```python
from build123d import *

# Parameters (mm, degrees)
F0_W     = 155.2556827664
F0_H     = 118.4387393296
F1_DEPTH = 57.1
F3_D     = 4.2
F4_R     = 5
F5_SIZE  = 5


with BuildPart() as f1:
    # F0 (on Front) → F1 (new body)
    with BuildSketch(Plane.XZ):
        with Locations((10.389957577, 21.1075376719)):
            Rectangle(F0_W, F0_H)
    extrude(amount=F1_DEPTH)

    # F3 (through all)
    with Locations(Plane(origin=(0, 0, 0), x_dir=(-1, 0, 0), z_dir=(0, 1, 0))):
        with Locations((-35.4269519448, 45.1725050807), (36.4308133721, 45.1725050807), (36.4308133721, 11.5158585832), (-35.4269519448, 11.5158585832)):
            Hole(F3_D / 2)

    # F4
    f4_edges = [f1.edges().sort_by_distance(p)[0] for p in [
        (-67.237884, -28.55, 80.326907),
    ]]
    fillet(f4_edges, radius=F4_R)

    # F5
    f5_edges = [f1.edges().sort_by_distance(p)[0] for p in [
        (88.017799, -28.55, 80.326907),
    ]]
    chamfer(f5_edges, length=F5_SIZE)


solid = f1.part
```
Here's how the part is built. I have some questions about the finished solid (model axes, mm). Coordinates: 2 decimals unless noted, no trailing zeros. Answer as CSV lines item,"result". Start each with the question number.
Q1. I need wall thicknesses on probe 1 along Z at (x, y) = (-35, -24.5). Which ranges of the line are inside material? Lowest first, please. Write a range as [from, to].
Q2. If we mould it in two halves opening along X, with no side actions, what happens to faces 1 (the cylindrical face through (34.972, -28.95, 43.122)), 2 (the flat face through (9, -57.1, 22)), 3 (the flat face through (-67.238, -28, 18)), 4 (the flat face through (88.018, -28, 18))? For each: pulls with the +X half, pulls with the -X half, needs draft (parallel to the pull), parting line crosses it, or undercut.
Q3. Will this pin go through, and if not, where does the flat tip stop? pin 1 Ø6 at (x, z) = (71.5, -5.5) entering from +Y.
Entries:
1,probe 1,"z = [-38.11, 9.98], [13.05, 43.64], [46.71, 80.33]"
2,face 1,"undercut"
2,face 2,"needs draft"
2,face 3,"pulls with the -X half"
2,face 4,"pulls with the +X half"
3,pin 1,"stops at y = 0"
